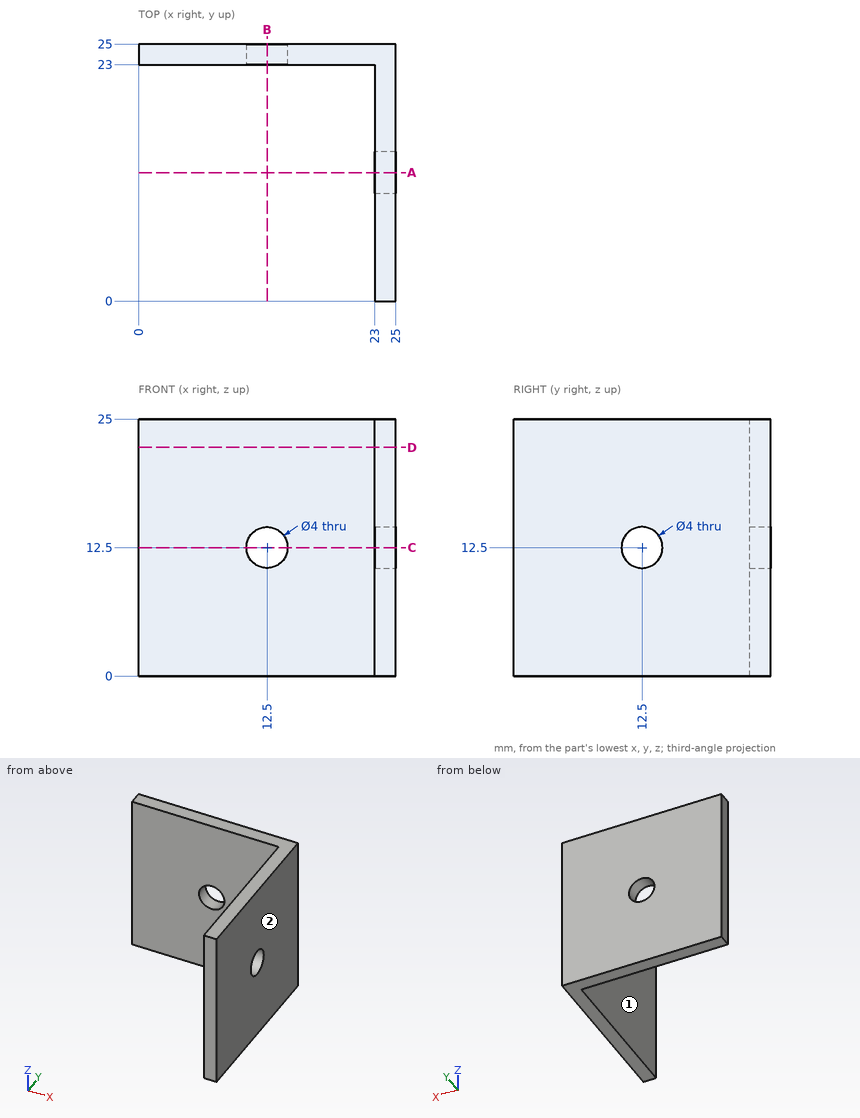
Verification items for this drawing (mm, ordinates from the low corner). A direction names the side the tool comes from. Round coordinates to 2 decimals unless told otherwise and drop trailing zeros. Order: outer loops, then holes, each group sorted by start corner. A loop starts at its lowest first (then second) coordinate and runs counter-clockwise, first axis right, second up. Notation, with made-up numbers: (-18, 11) - (-9, 11) arc R11 cw to (-9, 20) - close; hole circle Ø6 at (59, 20). An arc over 180 degrees is marked (long way). Answer as CSV lines item,"result". Start each with the question number.
1) Section check A-A (y = 12.5). Record the cut outline in (x, z).
2) Depth check by flat-ended pin: pin 1 (6.5 mm diameter, centred on x = 12.5, z = 12.5, fed in from +Y); pin 2 (11.5 mm diameter, centred on x = 9, z = 13, fed in from -Y); pin 3 (5 mm diameter, centred on y = 12.5, z = 12.5, fed in from -X). Enter the tip coordinate at first touch or a pass-through.
3) Section check D-D (z = 22.25). Record the cut outline in (x, y), then the cut area to 3 significant figures.
4) Section check C-C (z = 12.5). Record the cut outline in (x, y).
5) Scan lines: probe 1 along Z at (x, y) = (24.55, 12.5); probe 2 along Y at (x, z) = (6.5, 6). Record each from-to range of solid material in increasing order.
6) Tool access check on the marked faces 1 and 2. Record the directions out of +Z, -Z, +X, -X, +Y, -Y that give a thin tool (end or side, any length) a straight path to the whole face; none if there is none.
Determined:
1,outline,"(23, 0) - (25, 0) - (25, 10.5) - (23, 10.5) - close; (23, 14.5) - (25, 14.5) - (25, 25) - (23, 25) - close"
2,pin 1,"y = 25"
2,pin 2,"y = 23"
2,pin 3,"x = 23"
3,outline,"(0, 23) - (23, 23) - (23, 0) - (25, 0) - (25, 25) - (0, 25) - close"
3,area,"96.0 mm^2"
4,outline,"(0, 23) - (10.5, 23) - (10.5, 25) - (0, 25) - close; (14.5, 23) - (23, 23) - (23, 14.5) - (25, 14.5) - (25, 25) - (14.5, 25) - close; (23, 0) - (25, 0) - (25, 10.5) - (23, 10.5) - close"
5,probe 1,"0 to 10.5, 14.5 to 25"
5,probe 2,"23 to 25"
6,face 1,"+Z, -Z, -X, -Y"
6,face 2,"+Z, -Z, +X, +Y, -Y"
